Source: CAD feature listing. Evaluate the final solid. Frame: model axes, mm. Give positions to 0.01 mm unless a question says otherwise; leave off trailing zeros. Order: outer loops, then holes, each group sorted by start corner. A loop starts at its lowest first (then second) coordinate and runs counter-clockwise, first axis right, second up. Notation, with made-up numbers: (-21.5, 23) -> (20.5, 23) arc R20 cw to (20.5, 55) -> close; hole circle Ø4 at (1, 81). An arc over 180 degrees is marked (long way). Answer in a Markdown table with one row per item.
```python
from build123d import *

# Parameters (mm, degrees)
SKETCH1_W           = 15.9
SKETCH1_H           = 8
BOSS_EXTRUDE1_DEPTH = 20
SKETCH2_R           = 1.2
CUT_EXTRUDE1_DEPTH  = 16.9
SKETCH3_R           = 1.2
CUT_EXTRUDE2_DEPTH  = 9


with BuildPart() as part:
    # Sketch1 → Boss-Extrude1 (new body)
    with BuildSketch(Plane.XY):
        with Locations((7.95, 4)):
            Rectangle(SKETCH1_W, SKETCH1_H)
    extrude(amount=BOSS_EXTRUDE1_DEPTH)

    # Sketch2 → Cut-Extrude1 (cut, through all)
    with BuildSketch(Plane(origin=(15.9, 0, 0), x_dir=(0, 0, -1), z_dir=(1, 0, 0))):
        with Locations((-10, 3.5)):
            Circle(SKETCH2_R)
    extrude(amount=-CUT_EXTRUDE1_DEPTH, mode=Mode.SUBTRACT)

    # Sketch3 → Cut-Extrude2 (cut, through all)
    with BuildSketch(Plane(origin=(0, 8, 0), x_dir=(1, 0, 0), z_dir=(0, 1, 0))):
        with Locations((7.95, -15)):
            Circle(SKETCH3_R)
        with Locations((7.95, -5)):
            Circle(SKETCH3_R)
    extrude(amount=-CUT_EXTRUDE2_DEPTH, mode=Mode.SUBTRACT)


solid = part.part
```
(1) First-contact query: pin 1 Ø2 at (x, z) = (7.95, 5) entering from -Y. Flat tip, straight axial feed; report the tip coordinate or a pass-through.
A:
| item | result |
|---|---|
| pin 1 | passes through |
(2) Section query A-A (y = 3.5). Return the cut outline in (x, z), plus the area to 3 significant figures.
A:
| item | result |
|---|---|
| outline | (0, 0) -> (15.9, 0) -> (15.9, 8.8) -> (0, 8.8) -> close; (0, 11.2) -> (15.9, 11.2) -> (15.9, 20) -> (0, 20) -> close; hole circle Ø2.4 at (7.95, 5); hole circle Ø2.4 at (7.95, 15) |
| area | 271 mm^2 |
(3) Section query D-D (x = 12.25). Return the cut outline in (y, z), plus the area to 3 significant figures.
A:
| item | result |
|---|---|
| outline | (0, 0) -> (8, 0) -> (8, 20) -> (0, 20) -> close; hole circle Ø2.4 at (3.5, 10) |
| area | 155 mm^2 |
(4) Pull-direction query (Y, two-part tool) for faces 1 (the flat face through (8, 8, 10)), 2 (the cylindrical face through (8.06, 3.04, 8.89)), 3 (the cylindrical face through (6.75, 4.06, 4.95)); classes: +Y half, -Y half, draft (parallel to the pull), parting line (faces both ways), or undercut.
A:
| item | result |
|---|---|
| face 1 | +Y half |
| face 2 | undercut |
| face 3 | draft |
(5) Section query B-B (x = 7.95). Return the cut outline in (y, z), plus the area to 3 significant figures.
A:
| item | result |
|---|---|
| outline | (0, 0) -> (8, 0) -> (8, 3.8) -> (0, 3.8) -> close; (0, 6.2) -> (8, 6.2) -> (8, 13.8) -> (0, 13.8) -> close; (0, 16.2) -> (8, 16.2) -> (8, 20) -> (0, 20) -> close; hole circle Ø2.4 at (3.5, 10) |
| area | 117 mm^2 |
(6) Section query C-C (z = 5). Return the cut outline in (x, y), plus the area to 3 significant figures.
A:
| item | result |
|---|---|
| outline | (0, 0) -> (6.75, 0) -> (6.75, 8) -> (0, 8) -> close; (9.15, 0) -> (15.9, 0) -> (15.9, 8) -> (9.15, 8) -> close |
| area | 108 mm^2 |
(7) Ray query, probe 1 along Z at (x, y) = (7.95, 4.75); probe 2 along X at (y, z) = (4.25, 5); probe 3 along Y at (x, z) = (11, 10). Return the intervals inside material, ascending.
A:
| item | result |
|---|---|
| probe 1 | z = 0 to 3.8, 6.2 to 13.8, 16.2 to 20 |
| probe 2 | x = 0 to 6.75, 9.15 to 15.9 |
| probe 3 | y = 0 to 2.3, 4.7 to 8 |
